Autodesk Inventor part; units mm, degrees
ref_plane "YZ Plane" through (0, 0, 0) normal (1, 0, 0) x (0, 1, 0)
ref_plane "XZ Plane" through (0, 0, 0) normal (0, 1, 0) x (-1, 0, 0)
ref_plane "XY Plane" through (0, 0, 0) normal (0, 0, 1) x (1, 0, 0)
sketch "Sketch1" plane through (0, 0, 0) normal (0, 1, 0) x (-1, 0, 0)
  line L0 (445.6248, 255.5836) -> (415.6248, 255.5836)
  line L1 (415.6248, 255.5836) -> (415.6248, 235.5836)
  line L2 (415.6248, 235.5836) -> (445.6248, 235.5836)
  line L3 (445.6248, 235.5836) -> (445.6248, 255.5836)
  circle A0 centre (440.6248, 251.5836) radius 2.25
  circle A1 centre (440.6248, 239.5836) radius 2.25
  circle A2 centre (420.6248, 251.5836) radius 2.25
  circle A3 centre (420.6248, 239.5836) radius 2.25
  dimension "d8" = 4.5
  dimension "d9" = 20
  dimension "d10" = 30
  dimension "d11" = 20
  dimension "d12" = 12
  dimension "d13" = 4
  dimension "d14" = 5
extrude "Extrusion1" add sketch "Sketch1" along normal blind 5
fillet "Fillet1" radius 2 4 edges at (-415.6248, 2.5, 255.5836) (-415.6248, 2.5, 235.5836) (-445.6248, 2.5, 255.5836) (-445.6248, 2.5, 235.5836)
properties part number "beltpress"
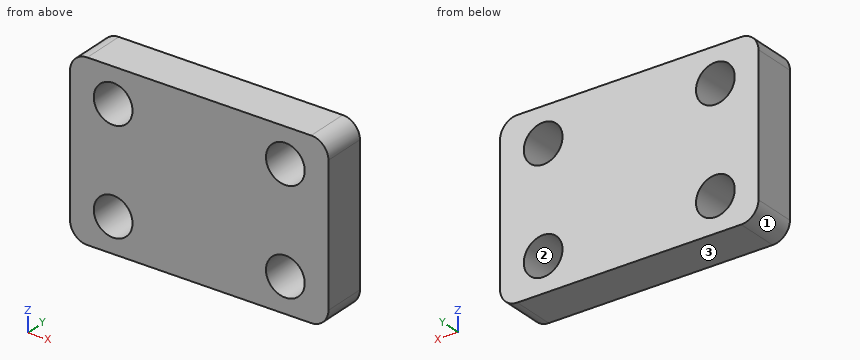
Model file for the job. Use its own axes, mm. Face numbers are marked on the shaded views. Coordinates: 2 decimals unless noted, no trailing zeros. Write each loop counter-clockwise with the first axis right and the second up, starting at its lowest first coordinate (ties: lowest second). Pieces come first, ordered by that corner, then holes. Notation, with made-up numbers: (68, 15.25) - (82, 15.25) arc R15 cw to (82, 37.25) - close; hole circle Ø1 at (9, 41.25). An arc over 180 degrees is marked (long way). Write each question's results on one line, items separated by ' | '. Start each with the question number.
1) Cut at A-A (x = -421.5). Write the cut outline in (y, z), then the cut area to 3 significant figures.
2) Cut at B-B (y = 1.7). Write the cut outline in (x, z).
3) Cut at C-C (z = 238.75). Write the cut outline in (x, y), then the cut area to 3 significant figures.
4) Mould opens along X. For the marked faces 1, 2 and 3 say: pulls with the +X half, pulls with the -X half, needs draft (parallel to the pull), parting line crosses it, or undercut.
5) Probe line 1 along Z through (x, y) = (-440.75, 2.35); line 2 along X through (y, z) = (1.55, 251.5); line 3 along X through (y, z) = (4, 251). List the from-to ranges inside material, lowest first. Write a range as from..to.
6) Flat gauge pin, fed straight in: P1, Ø2.5, axis at x = -440.62, z = 251.58, coming from the -Y side. Where does the tip first touch, or does it go through?
Returned:
1) outline: (0, 235.58) - (5, 235.58) - (5, 237.51) - (0, 237.51) - close; (0, 241.66) - (5, 241.66) - (5, 249.51) - (0, 249.51) - close; (0, 253.66) - (5, 253.66) - (5, 255.58) - (0, 255.58) - close | area: 58.5 mm^2
2) outline: (-445.62, 237.58) arc R2 ccw to (-443.62, 235.58) - (-417.62, 235.58) arc R2 ccw to (-415.62, 237.58) - (-415.62, 253.58) arc R2 ccw to (-417.62, 255.58) - (-443.62, 255.58) arc R2 ccw to (-445.62, 253.58) - close; hole circle Ø4.5 at (-440.62, 239.58); hole circle Ø4.5 at (-440.62, 251.58); hole circle Ø4.5 at (-420.62, 239.58); hole circle Ø4.5 at (-420.62, 251.58)
3) outline: (-445.62, 0) - (-442.71, 0) - (-442.71, 5) - (-445.62, 5) - close; (-438.53, 0) - (-422.71, 0) - (-422.71, 5) - (-438.53, 5) - close; (-418.53, 0) - (-415.62, 0) - (-415.62, 5) - (-418.53, 5) - close | area: 108 mm^2
4) face 1: pulls with the -X half | face 2: undercut | face 3: needs draft
5) line 1: 235.58..237.34, 241.83..249.34, 253.83..255.58 | line 2: -445.62..-442.87, -438.38..-422.87, -418.38..-415.62 | line 3: -445.62..-442.8, -438.45..-422.8, -418.45..-415.62
6) P1: through
